from build123d import *
from build123d.topology import SkipClean

# Parameters (mm, degrees)
SKETCH1_W                       = 44.069
SKETCH1_H                       = 16.8402
BOSS_EXTRUDE1_DEPTH             = 7.1628
SKETCH2_W                       = 26.3906
SKETCH2_H                       = 16.8402
CUT_EXTRUDE1_DEPTH              = 4.75
SKETCH4_W                       = 11.1887
SKETCH4_H                       = 1.5875
SKETCH4_W_2                     = 6.4897
CUT_EXTRUDE9_DEPTH              = 4.75
SKETCH5_R                       = 1.5875
CUT_EXTRUDE10_DEPTH             = 46.43435428
SKETCH14_W                      = 11.1887
SKETCH14_H                      = 13.6652
SKETCH14_W_2                    = 6.4897
BOSS_EXTRUDE3_DEPTH             = 1.5
SKETCH6_R                       = 0.889
CUT_EXTRUDE11_DEPTH             = 26.128895282
SKETCH7_R                       = 1.3208
CUT_EXTRUDE12_DEPTH             = 1.397
SKETCH9_R                       = 0.889
CUT_EXTRUDE13_DEPTH             = 26.128895282
SKETCH10_R                      = 1.190625
CUT_EXTRUDE14_DEPTH             = 1
CUT_EXTRUDE15_DEPTH             = 26.128895282
SKETCH12_R                      = 3.1115
CUT_EXTRUDE16_DEPTH             = 10.922
CUT_EXTRUDE16_DIRECTION_2_REACH = 37.029
BOSS_EXTRUDE4_START             = 3.5
BOSS_EXTRUDE4_DEPTH             = 3.5


with BuildPart() as part:
    # Sketch1 → Boss-Extrude1 (new body)
    with BuildSketch(Plane.XY):
        Rectangle(SKETCH1_W, SKETCH1_H)
    extrude(amount=BOSS_EXTRUDE1_DEPTH)

    # Sketch2 → Cut-Extrude1 (cut)
    with BuildSketch(Plane.XY.offset(7.1628)):
        with Locations((2.3495, 0)):
            Rectangle(SKETCH2_W, SKETCH2_H)
    extrude(amount=-CUT_EXTRUDE1_DEPTH, mode=Mode.SUBTRACT)

    # Sketch4 → Cut-Extrude9 (cut)
    with BuildSketch(Plane.XY.offset(7.1628)):
        with Locations((-16.44015, -7.62635)):
            Rectangle(SKETCH4_W, SKETCH4_H)
        with Locations((-16.44015, 7.62635)):
            Rectangle(SKETCH4_W, SKETCH4_H)
        with Locations((18.78965, -7.62635)):
            Rectangle(SKETCH4_W_2, SKETCH4_H)
        with Locations((18.78965, 7.62635)):
            Rectangle(SKETCH4_W_2, SKETCH4_H)
    extrude(amount=-CUT_EXTRUDE9_DEPTH, mode=Mode.SUBTRACT)

    # Sketch5 → Cut-Extrude10 (cut, through all)
    with BuildSketch(Plane.ZY.offset(22.0345)):
        with Locations((5.1628, -6.8326)):
            Circle(SKETCH5_R)
        with Locations((5.1628, 6.8326)):
            Circle(SKETCH5_R)
    extrude(amount=-CUT_EXTRUDE10_DEPTH, mode=Mode.SUBTRACT)

    # Sketch14 → Boss-Extrude3 (add)
    with BuildSketch(Plane.XY.offset(7.1628)):
        with Locations((-16.44015, 0)):
            Rectangle(SKETCH14_W, SKETCH14_H)
        with Locations((18.78965, 0)):
            Rectangle(SKETCH14_W_2, SKETCH14_H)
    extrude(amount=BOSS_EXTRUDE3_DEPTH)

    # Sketch6 → Cut-Extrude11 (cut, through all)
    with BuildSketch(Plane.XY.offset(8.6628)):
        with Locations((19.4945, 3.429)):
            Circle(SKETCH6_R)
        with Locations((19.4945, -3.429)):
            Circle(SKETCH6_R)
    cut_extrude11 = extrude(amount=-CUT_EXTRUDE11_DEPTH, mode=Mode.SUBTRACT)

    # Sketch7 → Cut-Extrude12 (cut)
    with BuildSketch(Plane.XY.offset(8.6628)):
        with Locations((19.4945, 3.429)):
            Circle(SKETCH7_R)
        with Locations(Location((19.4945, -3.429, 0), (0, 0, 180))):
            Circle(SKETCH7_R)
    cut_extrude12 = extrude(amount=-CUT_EXTRUDE12_DEPTH, mode=Mode.SUBTRACT)

    # Sketch9 → Cut-Extrude13 (cut, through all)
    with BuildSketch(Plane(origin=(0, 0, 0), x_dir=(-1, 0, 0), z_dir=(0, 0, -1))):
        with Locations((-2.3495, 5.4356)):
            Circle(SKETCH9_R)
        with Locations(Location((-2.3495, -5.4356, 0), (0, 0, 180))):
            Circle(SKETCH9_R)
    extrude(amount=-CUT_EXTRUDE13_DEPTH, mode=Mode.SUBTRACT)

    # Sketch10 → Cut-Extrude14 (cut)
    with BuildSketch(Plane(origin=(0, 0, 0), x_dir=(-1, 0, 0), z_dir=(0, 0, -1))):
        with Locations((-2.3495, 5.4356)):
            Circle(SKETCH10_R)
        with Locations(Location((-2.3495, -5.4356, 0), (0, 0, 180))):
            Circle(SKETCH10_R)
    extrude(amount=-CUT_EXTRUDE14_DEPTH, mode=Mode.SUBTRACT)

    # Sketch11 → Cut-Extrude15 (cut, through all)
    with BuildSketch(Plane(origin=(0, 0, 0), x_dir=(-1, 0, 0), z_dir=(0, 0, -1))):
        with BuildLine():
            Line((-11.3495, 3.75), (6.6505, 3.75))
            ThreePointArc((6.6505, 3.75), (10.4005, 0), (6.6505, -3.75))
            Line((6.6505, -3.75), (-11.3495, -3.75))
            ThreePointArc((-11.3495, -3.75), (-15.0995, 0), (-11.3495, 3.75))
        make_face()
    extrude(amount=-CUT_EXTRUDE15_DEPTH, mode=Mode.SUBTRACT)

    # Sketch12 → Cut-Extrude16 (cut)
    with BuildSketch(Plane(origin=(-10.8458, 0, 0), x_dir=(0, 0, -1), z_dir=(1, 0, 0))):
        with Locations(Location((-5.1628, 0, 0), (0, 0, 332.106408593))):
            Circle(SKETCH12_R)
    extrude(amount=-CUT_EXTRUDE16_DEPTH, mode=Mode.SUBTRACT)

    # Sketch12 → Cut-Extrude16 direction 2 (cut, up to next)
    with BuildSketch(Plane(origin=(-10.8458, 0, 0), x_dir=(0, 0, -1), z_dir=(1, 0, 0)), mode=Mode.PRIVATE) as cut_extrude16_direction_2_sk1:
        with Locations(Location((-5.1628, 0, 0), (0, 0, 332.106408593))):
            Circle(SKETCH12_R)
    cut_extrude16_direction_2_tool1 = extrude(cut_extrude16_direction_2_sk1.sketch, amount=CUT_EXTRUDE16_DIRECTION_2_REACH, mode=Mode.PRIVATE) & part.part
    add(cut_extrude16_direction_2_tool1.solids().sort_by_distance((-10.8458, 0, 5.1628))[0], mode=Mode.SUBTRACT)

    # Sketch15 → Boss-Extrude4 (add)
    with SkipClean():  # the faces are left unmerged after this step: merging them gives an invalid solid
        with BuildSketch(Plane.ZY.offset(22.0345).offset(BOSS_EXTRUDE4_START)):
            with BuildLine():
                Line((8.6628, 6.8326), (6.7503, 6.8326))
                ThreePointArc((6.7503, 6.8326), (5.1628, 5.2451), (3.5753, 6.8326))
                Line((3.5753, 6.8326), (2.4128, 6.8326))
                Line((2.4128, 6.8326), (2.4128, 8.4201))
                Line((2.4128, 8.4201), (0, 8.4201))
                Line((0, 8.4201), (0, -8.4201))
                Line((0, -8.4201), (2.4128, -8.4201))
                Line((2.4128, -8.4201), (2.4128, -6.8326))
                Line((2.4128, -6.8326), (3.5753, -6.8326))
                ThreePointArc((3.5753, -6.8326), (5.1628, -5.2451), (6.7503, -6.8326))
                Line((6.7503, -6.8326), (8.6628, -6.8326))
                Line((8.6628, -6.8326), (8.6628, 6.8326))
            make_face()
        extrude(amount=-BOSS_EXTRUDE4_DEPTH)
    add(part.part.scale(1), mode=Mode.REPLACE)  # the faces are merged on a copy

    # Mirror1: Cut-Extrude11, Cut-Extrude12 across plane
    add(cut_extrude11.mirror(Plane(origin=(-1.75, 0, 0), x_dir=(0, 0, 1), z_dir=(1, 0, 0))), mode=Mode.SUBTRACT)
    add(cut_extrude12.mirror(Plane(origin=(-1.75, 0, 0), x_dir=(0, 0, 1), z_dir=(1, 0, 0))), mode=Mode.SUBTRACT)


solid = part.part
Design review of the part built by this model. Coordinates are the model's own, in mm. A direction names the side the tool comes from. Round coordinates to 2 decimals unless told otherwise and drop trailing zeros. Write each loop counter-clockwise with the first axis right and the second up, starting at its lowest first coordinate (ties: lowest second). Pieces come first, ordered by that corner, then holes.
Item 1: Consider section B-B on z = 4.25. Give the boundary of the cut face in (x, y).
Item 2: Draft analysis for pull direction X (two halves, no side actions). For faces 1 (the cylindrical face through (-21.675, 3.487, 7.974)), 2 (the flat face through (-25.534, 0, 4)), 3 (the flat face through (19, 0, 8.663)), state which applies: released by +X, released by -X, zero draft, split by the parting line, or undercut.
Item 3: Consider section A-A on x = 7. Give the boundary of the cut face in (y, z).
Item 4: Wall thickness on L1, parallel to X at y = -3.5, z = 5.75; L2, parallel to X at y = -4.5, z = 6.5; L3, parallel to Y at x = 10, z = 2.25: over which ranges is each line inside the solid? List them lowest first.
Item 5: Consider section C-C on y = 0. Give the boundary of the cut face in (x, z), and give its area (3 significant figures).
Item 6: For pin 1 Ø1.5 at (x, z) = (18, 7.5) entering from +Y; pin 2 Ø2 at (x, y) = (2.35, 5.44) entering from +Z, all flat-tipped, find the tip position at first contact; note any pin that passes through.
Item 7: For faces 4 (the cylindrical face through (18.175, 3.487, 7.974)), 5 (the flat face through (-18, -6.833, 3)), 6 (the flat face through (-18, 6.833, 8)), 7 (the flat face through (15.545, 0, 6)), list the 3-axis set-ups (+Z, -Z, +X, -X, +Y, -Y) from which the entire face can be reached by the end or side of a thin tool; tool diameter is ignored.
Check values:
1. outline: (-25.53, -5.53) - (-10.85, -5.53) - (-10.85, -2.97) - (-21.77, -2.97) - (-21.77, 2.97) - (-10.85, 2.97) - (-10.85, 5.53) - (-25.53, 5.53) - close; (15.54, -5.53) - (22.03, -5.53) - (22.03, 5.53) - (15.54, 5.53) - close; hole circle Ø1.78 at (-22.99, -3.43); hole circle Ø1.78 at (-22.99, 3.43); hole circle Ø1.78 at (19.49, -3.43); hole circle Ø1.78 at (19.49, 3.43)
2. face 1: undercut
2. face 2: released by -X
2. face 3: zero draft
3. outline: (-8.42, 0) - (-3.75, 0) - (-3.75, 2.41) - (-8.42, 2.41) - close; (3.75, 0) - (8.42, 0) - (8.42, 2.41) - (3.75, 2.41) - close
4. L1: x = -25.53 to -23.88, -22.11 to -10.85, 15.54 to 18.61, 20.38 to 22.03
4. L2: x = -25.53 to -10.85, 15.54 to 22.03
4. L3: y = -8.42 to -3.75, 3.75 to 8.42
5. outline: (-25.53, 0) - (-10.4, 0) - (-10.4, 2.05) - (-21.77, 2.05) - (-21.77, 8.27) - (-10.85, 8.27) - (-10.85, 8.66) - (-25.53, 8.66) - close; (15.1, 0) - (22.03, 0) - (22.03, 8.66) - (15.54, 8.66) - (15.54, 2.41) - (15.1, 2.41) - close
5. area: 117 mm2
6. pin 1: stops at y = 6.83
6. pin 2: stops at z = 2.41
7. face 4: +Z
7. face 5: +Z, +X, -X, -Y
7. face 6: +Z, +X, -X, +Y
7. face 7: +Z, +Y, -Y
